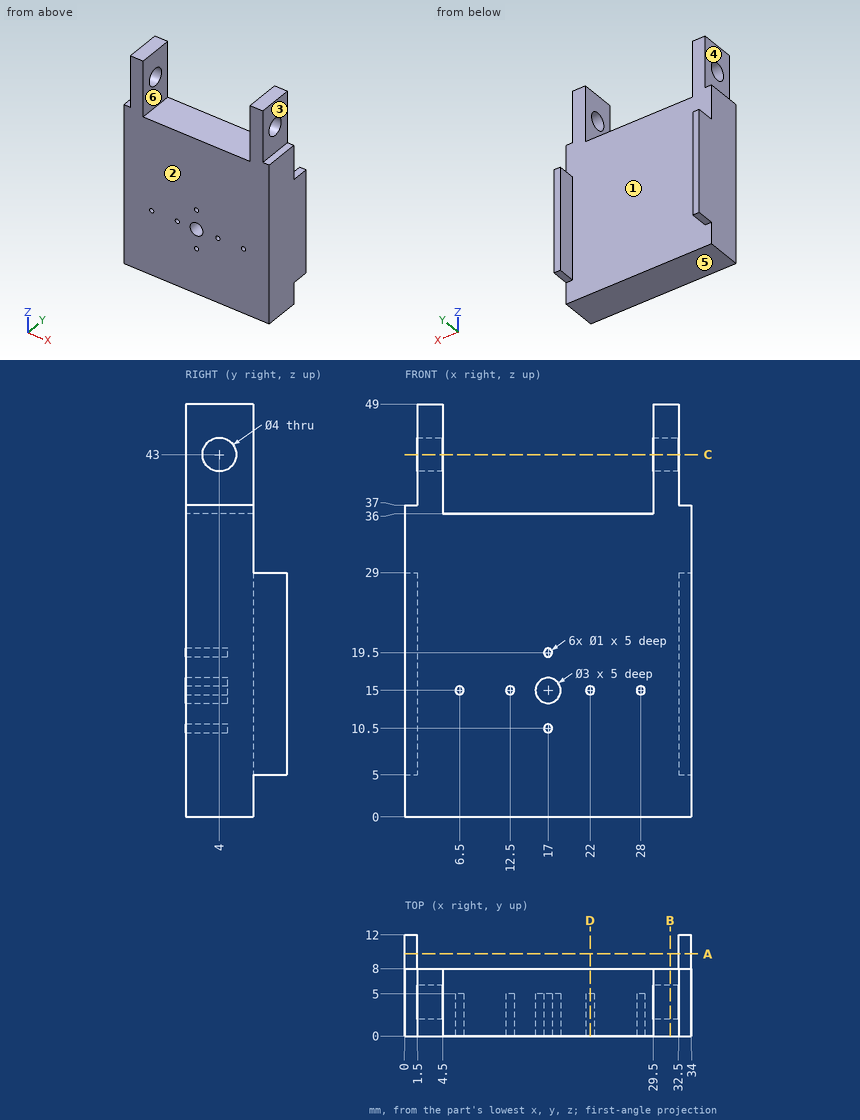
Verification items for this drawing (mm, ordinates from the low corner). A direction names the side the tool comes from. Give positions to 0.01 mm unless a question says otherwise; leave off trailing zeros. Loops run counter-clockwise (first coordinate to the right, second up) from the corner with the lowest first, then second, coordinate; pieces in that order, holes last. Notation, with made-up numbers: M -23,1 L 35,1 A16 cw 35,29 Z; hole C -27,9.25 d11. An arc over 180 degrees is marked long. Write item = value, one per line.
(1) Material ranges on line 1 (X direction, y = 0.5, z = 15); line 2 (Y direction, x = 4, z = 43); line 3 (X direction, y = 6.75, z = 42.5), recorded low to high. Write a range as [from, to].
Answer below:
line_1 = [0, 6], [7, 12], [13, 15.5], [18.5, 21.5], [22.5, 27.5], [28.5, 34]
line_2 = [0, 2], [6, 8]
line_3 = [1.5, 4.5], [29.5, 32.5]
(2) Sectioned sample at A-A, the plane y = 9.75. Record the cut outline in (x, z), plus the area to 3 significant figures.
Answer below:
outline = M 0,5 L 1.5,5 L 1.5,29 L 0,29 Z; M 32.5,5 L 34,5 L 34,29 L 32.5,29 Z
area = 72.0 mm2
(3) Gauge pin test, flat ends, axial feed: pin 1 Ø6 at (x, z) = (27.5, 20.5) entering from +Y; pin 2 Ø4 at (y, z) = (5.5, 43) entering from +X; pin 3 Ø2.5 at (y, z) = (4, 43) entering from +X; pin 4 Ø0.8 at (x, z) = (17, 19.5) entering from -Y. Record the tip position at first contact, or that the pin passes through.
Answer below:
pin_1 = 8
pin_2 = 32.5
pin_3 = through
pin_4 = 5
(4) Tool access check on the marked faces 5 and 6. Record the directions out of +Z, -Z, +X, -X, +Y, -Y that give a thin tool (end or side, any length) a straight path to the whole face; none if there is none.
Answer below:
face_5 = -Z, +X, -X, +Y, -Y
face_6 = +Z, +Y, -Y
(5) Sectioned sample at B-B, the plane x = 31.5. Record the cut outline in (y, z).
Answer below:
outline = M 0,0 L 8,0 L 8,49 L 0,49 Z; hole C 4,43 d4
(6) Release check for a two-part mould opening along X. For the marked faces 1, 2, 3 and 4 record: released by +X, released by -X, zero draft, split by the parting line, or undercut.
Answer below:
face_1 = undercut
face_2 = zero draft
face_3 = released by +X
face_4 = released by -X
(7) Sectioned sample at D-D, the plane x = 22. Record the cut outline in (y, z), plus the area to 3 significant figures.
Answer below:
outline = M 0,0 L 8,0 L 8,36 L 0,36 L 0,15.5 L 5,15.5 L 5,14.5 L 0,14.5 Z
area = 283 mm2
(8) Sectioned sample at C-C, the plane z = 43. Record the cut outline in (x, y).
Answer below:
outline = M 1.5,0 L 4.5,0 L 4.5,2 L 1.5,2 Z; M 1.5,6 L 4.5,6 L 4.5,8 L 1.5,8 Z; M 29.5,0 L 32.5,0 L 32.5,2 L 29.5,2 Z; M 29.5,6 L 32.5,6 L 32.5,8 L 29.5,8 Z
